from build123d import *

# Parameters (mm, degrees)
POCKET_DEPTH = 1.25


with BuildPart() as part:
    # Sketch (on DatumPlane) → Revolution (revolve)
    with BuildSketch(Plane.YZ):
        Polygon((0, 0), (0, -2.5), (19.75, -2.5), (20, -2.25), (20, -0.25), (19.75, 0), align=None)
    revolve(axis=Axis((0, 0, 0), (0, 0, 1)))

    # Sketch005 → Pocket (cut)
    with BuildSketch(Plane.XY):
        with BuildLine():
            add(Edge.make_bspline(
                [(-7.956615, 12.5), (-14.3, 7.725144)],
                knots=[0, 0, 42.868665, 42.868665], degree=1))
            add(Edge.make_bspline(
                [(-14.3, 7.725144), (-14.3, 0.021589)],
                knots=[0, 0, 41.594, 41.594], degree=1))
            add(Edge.make_bspline(
                [(-14.3, 0.021589), (0.047904, -16.207292)],
                knots=[0, 0, 116.959765, 116.959765], degree=1))
            add(Edge.make_bspline(
                [(0.047904, -16.207292), (14.407292, 0.021589)],
                knots=[0, 0, 117.00084, 117.00084], degree=1))
            add(Edge.make_bspline(
                [(14.407292, 0.021589), (14.407292, 7.725144)],
                knots=[0, 0, 41.594, 41.594], degree=1))
            add(Edge.make_bspline(
                [(14.407292, 7.725144), (8.063906, 12.5)],
                knots=[0, 0, 42.868665, 42.868665], degree=1))
            add(Edge.make_bspline(
                [(8.063906, 12.5), (0.047904, 7.181002)],
                knots=[0, 0, 51.942525, 51.942525], degree=1))
            add(Edge.make_bspline(
                [(0.047904, 7.181002), (-7.956615, 12.5)],
                knots=[0, 0, 51.890875, 51.890875], degree=1))
        make_face()
        with BuildLine():
            add(Edge.make_bspline(
                [(-8.205498, 9.386277), (-6.80486, 7.522711)],
                knots=[0, 0, 12.587107, 12.587107], degree=1))
            add(Edge.make_bspline(
                [(-6.80486, 7.522711), (-8.986799, 5.884766)],
                knots=[0, 0, 14.731081, 14.731081], degree=1))
            add(Edge.make_bspline(
                [(-8.986799, 5.884766), (-8.986799, 3.893776)],
                knots=[0, 0, 10.75, 10.75], degree=1))
            add(Edge.make_bspline(
                [(-8.986799, 3.893776), (-11.319313, 3.893776)],
                knots=[0, 0, 12.594, 12.594], degree=1))
            add(Edge.make_bspline(
                [(-11.319313, 3.893776), (-11.319313, 7.048059)],
                knots=[0, 0, 17.031, 17.031], degree=1))
            add(Edge.make_bspline(
                [(-11.319313, 7.048059), (-8.20559, 9.386315)],
                knots=[0, 0, 21.024604, 21.024604], degree=1))
            add(Edge.make_bspline(
                [(-8.20559, 9.386315), (-8.205498, 9.386277)],
                knots=[0, 0, 0.000539, 0.000539], degree=1))
        make_face(mode=Mode.SUBTRACT)
    extrude(amount=-POCKET_DEPTH, mode=Mode.SUBTRACT)


solid = part.part
Work out the finished part from the listing and answer in its coordinate system (mm). Coordinates: 2 decimals unless noted, no trailing zeros. Answer as CSV lines item,"result". Start each with the question number.
Item 1: Consider L1, parallel to X at y = 7.5, z = -1.1; L2, parallel to X at y = 11, z = -0.5; L3, parallel to Y at x = -8, z = -0.2. Determine where each line is inside the solid, lowest interval first.
Item 2: Flat-ended cylindrical pins translate along their axes: P1, Ø5, axis at x = -0.5, y = 4.5, coming from the +Z side; P2, Ø1.5, axis at x = 6.5, z = -2, coming from the -Y side; P3, Ø1.5, axis at y = 0, z = -2, coming from the +X side. Find the tip coordinate at first contact, or state that the pin passes through.
Item 3: Determine the mould class of faces 1 (the face through (0, 2, -1.25)), 2 (the face through (0, 0, -2.5)), 3 (the face through (19.524, -4.336, -1.236)) for opening direction Y: released by +Y, released by -Y, zero draft, split by the parting line, or undercut.
Item 4: Section A-A on z = -0.75 is taken. Give the number of separate pieces and of enclosed holes in the cut face, and give its area (3 significant figures).
Checks:
1,L1,"x = -18.54 to -14.3, -10.72 to -6.84, -0.43 to 0.53, 14.41 to 18.54"
1,L2,"x = -16.7 to -9.95, -5.7 to 5.8, 10.06 to 16.7"
1,L3,"y = -18.28 to -7.1, 6.63 to 9.11, 12.47 to 18.28"
2,P1,"stops at z = -1.25"
2,P2,"stops at y = -19.16"
2,P3,"stops at x = 20"
3,face 1,"undercut"
3,face 2,"zero draft"
3,face 3,"split by the parting line"
4,separate pieces,"2"
4,enclosed holes,"1"
4,area,"752 mm²"
